The listing builds one solid part. Answer for the finished solid, in the listing's coordinates (mm). Face numbers are marked on the shaded views. Give positions to 0.01 mm unless a question says otherwise; leave off trailing zeros. Write each loop counter-clockwise with the first axis right and the second up, starting at its lowest first coordinate (ties: lowest second). Pieces come first, ordered by that corner, then holes. Notation, with made-up numbers: (44.25, -6.5) - (57.25, -6.5) arc R7 ccw to (57.25, -2.5) - close; hole circle Ø5 at (10, 4.25). An arc over 180 degrees is marked (long way). Return JSON: item names as keys, results as strings.
from build123d import *

# Parameters (mm, degrees)
SKETCH1_R           = 4.9
BOSS_EXTRUDE1_DEPTH = 100
CUT_EXTRUDE1_DEPTH  = 10


with BuildPart() as part:
    # Sketch1 → Boss-Extrude1 (new body)
    with BuildSketch(Plane.YZ):
        with Locations(Location((0, 0, 0), (0, 0, 270))):
            Circle(SKETCH1_R)
    extrude(amount=BOSS_EXTRUDE1_DEPTH)

    # Sketch2 → Cut-Extrude1 (cut)
    with BuildSketch(Plane(origin=(0, 0, 0), x_dir=(0, -1, 0), z_dir=(-1, 0, 0))):
        with BuildLine():
            Line((-1.85, -1.280624847), (-1.85, 1.280624847))
            ThreePointArc((-1.85, 1.280624847), (0, 2.25), (1.85, 1.280624847))
            Line((1.85, 1.280624847), (1.85, -1.280624847))
            ThreePointArc((1.85, -1.280624847), (0, -2.25), (-1.85, -1.280624847))
        make_face()
    extrude(amount=-CUT_EXTRUDE1_DEPTH, mode=Mode.SUBTRACT)


solid = part.part
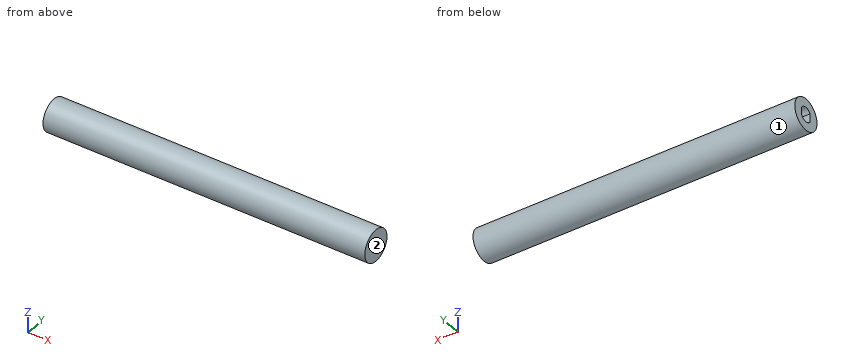
Item 1: The mould has two halves that part along X. Classify the marked faces 1 and 2: +X half, -X half, draft (parallel to the pull), parting line (faces both ways), or undercut.
Answer below:
{"face 1": "draft", "face 2": "+X half"}
Item 2: A cutting plane is placed at B-B on z = 0. Determine the outline of the cut face in (x, y), then the cut area to 3 significant figures.
Answer below:
{"outline": "(0, -4.9) - (100, -4.9) - (100, 4.9) - (0, 4.9) - (0, 1.85) - (10, 1.85) - (10, -1.85) - (0, -1.85) - close", "area": "943 mm²"}
Item 3: Consider L1, parallel to Z at x = 52.5, y = 0.25; L2, parallel to X at y = 0.75, z = -1.25. Determine where each line is inside the solid, lowest interval first.
Answer below:
{"L1": "z = -4.89 to 4.89", "L2": "x = 10 to 100"}
Item 4: A cutting plane is placed at C-C on x = 49. Determine the outline of the cut face in (y, z), then the cut area to 3 significant figures.
Answer below:
{"outline": "circle Ø9.8 at (0, 0)", "area": "75.4 mm²"}
Item 5: A cutting plane is placed at A-A on y = 0. Determine the outline of the cut face in (x, z).
Answer below:
{"outline": "(0, -4.9) - (100, -4.9) - (100, 4.9) - (0, 4.9) - (0, 2.25) - (10, 2.25) - (10, -2.25) - (0, -2.25) - close"}
Item 6: Flat-ended cylindrical pins translate along their axes: P1, Ø3, axis at x = 43.5, z = -3, coming from the -Y side; P2, Ø1.5, axis at x = 12.5, z = -3.5, coming from the +Y side; P3, Ø1, axis at x = 53, y = 4, coming from the +Z side. Find the tip coordinate at first contact, or state that the pin passes through.
Answer below:
{"P1": "stops at y = -4.66", "P2": "stops at y = 4.06", "P3": "stops at z = 3.43"}
